from build123d import *

# Parameters (mm, degrees)
BOSS_EXTRUDE1_DEPTH    = 72
CONVERT_SOLID1_DEPTH   = 72
CONVERT_SOLID1_2_DEPTH = 72


# Read off the part's stored shape, not the designer's step: Convert-Solid1
with BuildPart() as part:
    # Sketch1 → Boss-Extrude1 (new body)
    with BuildSketch(Plane.XY):
        Polygon((0, 15), (0, 0), (10, 0), (10, 3.175), (3.175, 3.175), (3.175, 15), align=None)
    extrude(amount=BOSS_EXTRUDE1_DEPTH)

    # Convert-Solid1 outline → Convert-Solid1 (cut)
    with BuildSketch(Plane.XY):
        with BuildLine():
            Line((1.675, 5.175), (1.675, 15))
            Line((1.675, 15), (0, 15))
            Line((0, 15), (0, 0))
            Line((0, 0), (10, 0))
            Line((10, 0), (10, 1.675))
            Line((10, 1.675), (5.175, 1.675))
            ThreePointArc((5.175, 1.675), (2.700126266, 2.700126266), (1.675, 5.175))
        make_face()
    extrude(amount=CONVERT_SOLID1_DEPTH, mode=Mode.SUBTRACT)

    # Convert-Solid1 2 outline → Convert-Solid1 2 (add)
    with BuildSketch(Plane.XY):
        with BuildLine():
            ThreePointArc((5.175, 3.175), (3.760786438, 3.760786438), (3.175, 5.175))
            Line((3.175, 5.175), (3.175, 3.175))
            Line((3.175, 3.175), (5.175, 3.175))
        make_face()
    extrude(amount=CONVERT_SOLID1_2_DEPTH)


solid = part.part
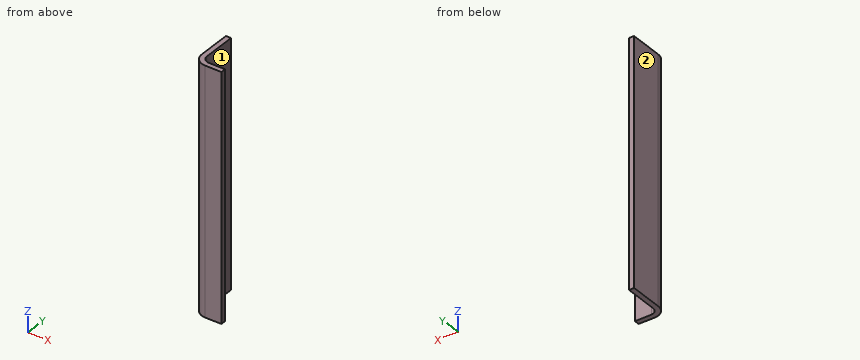
Design review of the part built by this model. Coordinates are the model's own, in mm. Face numbers are marked on the shaded views. A direction names the side the tool comes from. Coordinates: 2 decimals unless noted, no trailing zeros. Loops run counter-clockwise (first coordinate to the right, second up) from the corner with the lowest first, then second, coordinate; pieces in that order, holes last. Notation, with made-up numbers: M 41.5,60.5 L 62.5,60.5 A13 cw 62.5,84.5 Z; hole C 15.25,-30.5 d2. An arc over 180 degrees is marked long. Use one line per item in the form item = value.
(1) Clearance check with flat-ended pins moving along their axes: P1, Ø5, axis at y = 9, z = 21.5, coming from the +X side (3 decimals); P2, Ø3, axis at x = 2.5, z = 44, coming from the -Y side. State where each tip first meets the part, or that it passes through.
Return value:
P1 = 3.175
P2 = 1.88
(2) For line 1 along X through (y, z) = (6.75, 18.5) (3 decimals); line 2 along Y through (x, z) = (5, 31.5); line 3 along X through (y, z) = (3.75, 33), list the stretches that pass through material, from the lowest coordinate up. Write a range as from..to.
Return value:
line_1 = 1.675..3.175
line_2 = 1.68..3.18
line_3 = 1.98..3.77
(3) Consider section A-A (z = 53.5). Write out the cut boundary in (x, y) (3 decimals).
Return value:
outline = M 1.675,5.175 A3.5 ccw 5.175,1.675 L 10,1.675 L 10,3.175 L 5.175,3.175 A2 cw 3.175,5.175 L 3.175,15 L 1.675,15 Z
(4) For the marked faces 1 and 2, list the 3-axis set-ups (+Z, -Z, +X, -X, +Y, -Y) from which the entire face can be reached by the end or side of a thin tool; tool diameter is ignored.
Return value:
face_1 = +Z, -Z, +X, +Y
face_2 = +Z, -Z, -X, +Y, -Y
(5) Consider section B-B (y = 12.5). Write out the cut boundary in (x, z) (3 decimals), and give its area (3 significant figures).
Return value:
outline = M 1.675,0 L 3.175,0 L 3.175,72 L 1.675,72 Z
area = 108 mm2
